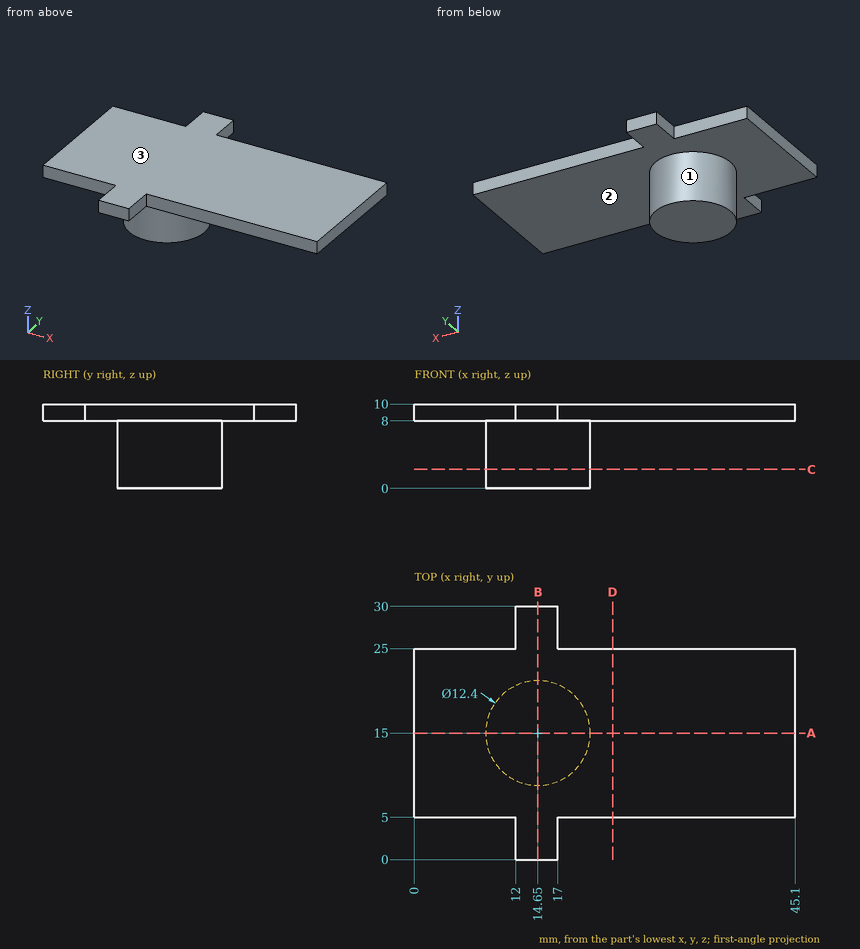
Input: dimensioned drawing with shaded views. Units: mm. Origin: part minimum x, y, z. Give positions to 0.01 mm unless a question says otherwise; leave off trailing zeros. Write each loop counter-clockwise with the first axis right and the second up, starting at its lowest first coordinate (ties: lowest second). Pieces come first, ordered by that corner, then holes. Notation, with made-up numbers: (22, 29.5) -> (51, 29.5) arc R23 ccw to (51, 65.5) -> close; hole circle Ø8 at (77, 16.5). An arc over 180 degrees is marked (long way). Return JSON: item names as keys, results as strings. Group by question number.
1. Mould query, pull axis Z, two halves, no side actions, for the marked faces 1, 2 and 3. Classes: +Z half, -Z half, draft (parallel to the pull), parting line (faces both ways), or undercut.
2. Material intervals for line 1 (Z direction, x = 2.5, y = 20.5); line 2 (Y direction, x = 14.5, z = 7); line 3 (X direction, y = 12, z = 3.5), sorted ascending. Write a range as from..to.
3. Section B-B, the plane x = 14.65. Output: boundary loops of the cut face in (y, z), then the cut area to 3 significant figures.
4. Section A-A, the plane y = 15. Output: boundary loops of the cut face in (x, z), then the cut area to 3 significant figures.
5. Section D-D, the plane x = 23.5. Output: boundary loops of the cut face in (y, z), then the cut area to 3 significant figures.
6. Section C-C, the plane z = 2.25. Output: boundary loops of the cut face in (x, y).
7. Pin query (flat end, axial travel): pin 1 Ø5 at (y, z) = (11.5, 2) entering from -X; pin 2 Ø2 at (y, z) = (2, 9) entering from +X; pin 3 Ø2 at (y, z) = (12, 6.5) entering from -X. Return the tip coordinate at first contact, or that it passes through.
Determined:
{
 "1": {"face 1": "draft", "face 2": "-Z half", "face 3": "+Z half"},
 "2": {"line 1": "z = 8..10", "line 2": "y = 8.8..21.2", "line 3": "x = 9.22..20.08"},
 "3": {"outline": "(0, 8) -> (8.8, 8) -> (8.8, 0) -> (21.2, 0) -> (21.2, 8) -> (30, 8) -> (30, 10) -> (0, 10) -> close", "area": "159 mm2"},
 "4": {"outline": "(0, 8) -> (8.45, 8) -> (8.45, 0) -> (20.85, 0) -> (20.85, 8) -> (45.1, 8) -> (45.1, 10) -> (0, 10) -> close", "area": "189 mm2"},
 "5": {"outline": "(5, 8) -> (25, 8) -> (25, 10) -> (5, 10) -> close", "area": "40.0 mm2"},
 "6": {"outline": "circle Ø12.4 at (14.65, 15)"},
 "7": {"pin 1": "stops at x = 8.53", "pin 2": "stops at x = 17", "pin 3": "stops at x = 8.78"}
}
